```python
from build123d import *

# Parameters (mm, degrees)
F1_DEPTH = 3
F2_R     = 1.5
F3_DEPTH = 25
F4_R     = 1.5
F5_DEPTH = 25
F6_W     = 121
F6_H     = 76
F6_R     = 1.5
F7_DEPTH = 3
F8_W     = 25
F8_H     = 24.5
F9_DEPTH = 3


# Not quite as in the source:
# - a feature names something its author has since deleted; it is built from what else it names


with BuildPart() as f1:
    # F0 (on Front) → F1 (new body)
    with BuildSketch(Plane.XZ):
        with BuildLine():
            Line((-75, -60), (75, -60))
            ThreePointArc((75, -60), (78.5355339059, -58.5355339059), (80, -55))
            Line((80, -55), (80, 55))
            ThreePointArc((80, 55), (78.5355339059, 58.5355339059), (75, 60))
            Line((75, 60), (-75, 60))
            ThreePointArc((-75, 60), (-78.5355339059, 58.5355339059), (-80, 55))
            Line((-80, 55), (-80, -55))
            ThreePointArc((-80, -55), (-78.5355339059, -58.5355339059), (-75, -60))
        make_face()
    extrude(amount=F1_DEPTH)

    # F2 (on Front) → F3 (cut)
    with BuildSketch(Plane.XZ):
        with Locations((-75, 55)):
            Circle(F2_R)
        with Locations((75, 55)):
            Circle(F2_R)
        with Locations((75, -55)):
            Circle(F2_R)
        with Locations((-75, -55)):
            Circle(F2_R)
    extrude(amount=F3_DEPTH, mode=Mode.SUBTRACT)

    # F4 (on Front) → F5 (cut)
    with BuildSketch(Plane.XZ):
        with Locations((52.5, 34.4)):
            Circle(F4_R)
    extrude(amount=F5_DEPTH, mode=Mode.SUBTRACT)

    # F6 (on face) → F7 (cut)
    with BuildSketch(Plane.XZ.offset(3)):
        with Locations((-4, -7.6)):
            Rectangle(F6_W, F6_H)
        with Locations((52.5, 34.4)):
            Circle(F6_R)
        with Locations((-60.5, 34.4)):
            Circle(F6_R)
        with Locations((-60.5, -49.6)):
            Circle(F6_R)
        with Locations((52.5, -49.6)):
            Circle(F6_R)
    extrude(amount=-F7_DEPTH, mode=Mode.SUBTRACT)

    # F8 (on face) → F9 (cut)
    with BuildSketch(Plane.XZ.offset(3)):
        with Locations((37.5, 42.65)):
            Rectangle(F8_W, F8_H)
    extrude(amount=-F9_DEPTH, mode=Mode.SUBTRACT)


solid = f1.part
```
The listing builds one solid part. Answer for the finished solid, in the listing's coordinates (mm). Coordinates: 2 decimals unless noted, no trailing zeros. Order: outer loops, then holes, each group sorted by start corner. A loop starts at its lowest first (then second) coordinate and runs counter-clockwise, first axis right, second up. Notation, with made-up numbers: M -37,-6 L -13,-6 A17 ccw -13,20 Z; hole C 21,1.5 d6. An arc over 180 degrees is marked long. Answer as a JSON object with one key per item and string values. Group by question number.
1. Section A-A on z = -37.5 is taken. Write down the section's boundary in (x, y).
2. Section B-B on y = -1.7 is taken. State how many separate pieces and enclosed holes the cut face has, then the cut area to 3 significant figures.
3. Straight lines are drawn through the part: line 1 (Z direction, x = 75, y = -1.4); line 2 (Z direction, x = 52.5, y = -1.4); line 3 (X direction, y = -0.5, z = 15.5). For each, find the intervals that lie inside material, in ascending order.
4. A flat-ended cylindrical pin translates along its axis: P1, Ø1.8, axis at x = -60.5, z = -49.6, coming from the -Y side. Find the tip coordinate at first contact, or state that the pin passes through.
5. Section C-C on x = -47 is taken. Write down the section's boundary in (y, z), then the cut area to 3 significant figures.
Values follow:
{
 "1": {"outline": "M -80,-3 L -64.5,-3 L -64.5,0 L -80,0 Z; M 56.5,-3 L 80,-3 L 80,0 L 56.5,0 Z"},
 "2": {"separate pieces": "1", "enclosed holes": "9", "area": "9,310 mm2"},
 "3": {"line 1": "-60 to -56.5, -53.5 to 53.5, 56.5 to 60", "line 2": "-60 to -51.1, -48.1 to -45.6, 30.4 to 32.9, 35.9 to 60", "line 3": "-80 to -64.5, 56.5 to 80"},
 "4": {"P1": "through"},
 "5": {"outline": "M -3,-60 L 0,-60 L 0,-45.6 L -3,-45.6 Z; M -3,30.4 L 0,30.4 L 0,60 L -3,60 Z", "area": "132 mm2"}
}
